```python
from build123d import *

# Parameters (mm, degrees)
F0_W     = 69.4388896227
F0_H     = 40.5697822571
F1_DEPTH = 181.864
F3_DEPTH = 80.01
F4_DEPTH = 105.41
F5_W     = 103.1131744385
F5_H     = 31.7430943251
F6_DEPTH = 25.4


# Not quite as in the source:
# - the program builds the solid bodies; features that only make, move or delete a surface that nothing else refers to are left out


with BuildPart() as f1:
    # F0 (on Front) → F1 (new body)
    with BuildSketch(Plane.XZ):
        with Locations((34.7194448113, 20.2848911285)):
            Rectangle(F0_W, F0_H)
    extrude(amount=F1_DEPTH)

    # F3 (add): a face of the model
    f3_faces = [f1.faces().sort_by_distance(p)[0] for p in [
        (34.7194448113, -90.932, 40.5697822571),
    ]]
    extrude(f3_faces, amount=F3_DEPTH)

    # F4 (add): a face of the model
    f4_faces = [f1.faces().sort_by_distance(p)[0] for p in [
        (34.7194448113, -181.864, 60.2898911285),
    ]]
    extrude(f4_faces, amount=F4_DEPTH)

    # F5 (on face) → F6 (join)
    with BuildSketch(Plane.YZ.offset(69.4388896227)):
        with Locations((-142.2493308783, 52.7632534504)):
            Rectangle(F5_W, F5_H)
    extrude(amount=F6_DEPTH)


solid = f1.part
```
Can you work these out from the model? Positions are in its coordinate system, mm. A direction names the side the tool comes from. Coordinates: 2 decimals unless noted, no trailing zeros. Order: outer loops, then holes, each group sorted by start corner. A loop starts at its lowest first (then second) coordinate and runs counter-clockwise, first axis right, second up.
1. If we section it at A-A (z = 61): Please give me the cut outline in (x, y), then the cut area to 3 significant figures.
2. Thinking about a two-plate mould opening in Y: for faces 1 (the face through (94.839, -143, 53)), 2 (the face through (34, -287.274, 59)), 3 (the face through (82, -90.693, 53)), which applies, +Y half, -Y half, draft (parallel to the pull), parting line (faces both ways), or undercut?
3. If we section it at C-C (x = 84): Please give me the cut outline in (y, z).
4. For faces 4 (the face through (82, -143, 68.635)), 5 (the face through (82, -143, 36.892)), 6 (the face through (82, -193.806, 53)), which set-ups out of +Z, -Z, +X, -X, +Y, -Y let a thin tool reach every point of the face, with its end or its side?
5. I need wall thicknesses on line 1 (Z direction, x = 75, y = -173); line 2 (X direction, y = -224, z = 55); line 3 (Y direction, x = 85.5, z = 63.5). Which ranges of each line are inside material? Lowest first, please.
6. If we section it at B-B (y = -70): Please give me the cut outline in (x, z).
7. I'm going to push flat-ended pins straight in: pin 1 (12.5 mm diameter, centred on x = 85, y = -134.5, fed in from +Z); pin 2 (2 mm diameter, centred on y = -171.5, z = 21.5, fed in from +X); pin 3 (20.5 mm diameter, centred on x = 82, z = 57.5, fed in from -Y). Where does each tip first touch, or does it pass through?
Entries:
1. outline: (0, -287.27) - (69.44, -287.27) - (69.44, -193.81) - (94.84, -193.81) - (94.84, -90.69) - (69.44, -90.69) - (69.44, 0) - (0, 0) - close
1. area: 22,600 mm2
2. face 1: draft
2. face 2: -Y half
2. face 3: +Y half
3. outline: (-193.81, 36.89) - (-90.69, 36.89) - (-90.69, 68.63) - (-193.81, 68.63) - close
4. face 4: +Z, +X, +Y, -Y
4. face 5: -Z, +X, +Y, -Y
4. face 6: +Z, -Z, +X, -Y
5. line 1: z = 36.89 to 68.63
5. line 2: x = 0 to 69.44
5. line 3: y = -193.81 to -90.69
6. outline: (0, 0) - (69.44, 0) - (69.44, 120.58) - (0, 120.58) - close
7. pin 1: stops at z = 68.63
7. pin 2: stops at x = 69.44
7. pin 3: stops at y = -193.81
